Verification items for the finished model (mm, model axes). A direction names the side the tool comes from. Coordinates: 2 decimals unless noted, no trailing zeros. Order: outer loops, then holes, each group sorted by start corner. A loop starts at its lowest first (then second) coordinate and runs counter-clockwise, first axis right, second up. Notation, with made-up numbers: M -7.5,-0.75 L 37.5,-0.75 A33 cw 37.5,28.25 Z; hole C 77,5 d2. An arc over 180 degrees is marked long. Return JSON: item names as keys, results as strings. Group by question number.
Q1. Section check B-B, the plane x = 0. Enter the section's corners in (y, z).
Q2. Mould release check, pull along Z, two halves, no side actions. Record for faces 1 (the face through (-10.4, 10.922, -6.3)), 2 (the face through (-9.37, 15.93, -7.19)), 3 (the face through (0, 11, 2.699)): pulls with the +Z half, pulls with the -Z half, needs draft (parallel to the pull), parting line crosses it, or undercut.
Q3. Thickness scan on probe 1 along Z at (x, y) = (0, 1.95); probe 2 along X at (y, z) = (2.75, -13); probe 3 along Y at (x, z) = (11.5, -20.5). Record the ranges inside material, lowest first.
Q4. Section check C-C, the plane y = 1.5. Enter the section's corners in (x, z), then the cut area to 3 significant figures.
Q5. Section check D-D, the plane x = 13. Enter the section's corners in (y, z), then the cut area to 3 significant figures.
Q6. Access from +Z, -Z, +X, -X, +Y, -Y to the whole of each face (thin tool, end or side, straight path). Record for faces 4 (the face through (0, 21.082, -3)), 5 (the face through (-1.82, 7.96, 13.85)), 6 (the face through (0, 11, -2.699)).
Q7. Go/stop test with flat-tipped pins: pin 1 Ø6.5 at (x, z) = (-20.62, -11.91) entering from +Y; pin 2 Ø3 at (y, z) = (10.5, 9) entering from +X; pin 3 Ø5 at (y, z) = (9, 2) entering from +X. Record where each tip stops, or that it passes through.
Q8. Section check A-A, the plane y = 5.75. Enter the section's corners in (x, z).
Autodesk Inventor part; units mm, degrees
ref_plane "YZ Plane" through (0, 0, 0) normal (1, 0, 0) x (0, 1, 0)
ref_plane "XZ Plane" through (0, 0, 0) normal (0, 1, 0) x (-1, 0, 0)
ref_plane "XY Plane" through (0, 0, 0) normal (0, 0, 1) x (1, 0, 0)
sketch "Sketch1" plane through (0, 0, 0) normal (0, 1, 0) x (-1, 0, 0)
  circle A0 centre (0, 0) radius 27.94
  dimension "d0" = 55.88
extrude "Extrusion1" add sketch "Sketch1" along normal blind 5.08
sketch "Sketch2" plane through (0, 5.08, 0) normal (0, 1, 0) x (1, 0, 0)
  circle A0 centre (0, 0) radius 13.97
  dimension "d3" = 27.94
extrude "Extrusion2" add sketch "Sketch2" along normal blind 5.842
sketch "Sketch3" plane through (0, 10.922, 0) normal (0, 1, 0) x (1, 0, 0)
  circle A0 centre (0, 0) radius 11.811
  dimension "d6" = 23.622
extrude "Extrusion3" add sketch "Sketch3" along normal blind 10.16
sketch "Sketch5" plane through (0, 21.082, 0) normal (0, 1, 0) x (1, 0, 0)
  line L0 (0, 0) -> (0, 2.667)
  line L1 (-3.1168, 0) -> (-1.5584, 2.6992)
  line L2 (-1.5584, 2.6992) -> (1.5584, 2.6992)
  line L3 (1.5584, 2.6992) -> (3.1168, 0)
  line L4 (3.1168, 0) -> (1.5584, -2.6992)
  line L5 (1.5584, -2.6992) -> (-1.5584, -2.6992)
  line L6 (-1.5584, -2.6992) -> (-3.1168, 0)
  dimension "d10" = 2.667
extrude "Extrusion4" cut sketch "Sketch5" against normal blind 25.4
sketch "Sketch6" plane through (0, 5.08, 0) normal (0, 1, 0) x (1, 0, 0)
  circle A0 centre (0, 0) radius 27.94
  circle A1 centre (0, 23.8125) radius 1.9939
  circle A2 centre (20.6222, 11.9063) radius 1.9939
  circle A3 centre (20.6222, -11.9063) radius 1.9939
  circle A4 centre (0, -23.8125) radius 1.9939
  circle A5 centre (-20.6222, -11.9063) radius 1.9939
  circle A6 centre (-20.6222, 11.9063) radius 1.9939
extrude "Extrusion5" cut sketch "Sketch6" against normal blind 25.4 contours A1 | A2 | A3 | A4 | A5 | A6
properties part number "Wheel Mount"
Numbers:
{
 "1": {"outline": "M 0,-27.94 L 5.08,-27.94 L 5.08,-25.81 L 0,-25.81 Z; M 0,-21.82 L 5.08,-21.82 L 5.08,-13.97 L 10.92,-13.97 L 10.92,-11.81 L 21.08,-11.81 L 21.08,-2.7 L 0,-2.7 Z; M 0,2.7 L 21.08,2.7 L 21.08,11.81 L 10.92,11.81 L 10.92,13.97 L 5.08,13.97 L 5.08,21.82 L 0,21.82 Z; M 0,25.81 L 5.08,25.81 L 5.08,27.94 L 0,27.94 Z"},
 "2": {"face 1": "needs draft", "face 2": "parting line crosses it", "face 3": "undercut"},
 "3": {"probe 1": "z = -27.94 to -25.81, -21.82 to -2.7, 2.7 to 21.82, 25.81 to 27.94", "probe 2": "x = -24.73 to -22.29, -18.96 to 18.96, 22.29 to 24.73", "probe 3": "y = 0 to 5.08"},
 "4": {"outline": "C 0,0 d55.88; hole C -20.62,-11.91 d3.99; hole C -20.62,11.91 d3.99; hole M -3.12,0 L -1.56,-2.7 L 1.56,-2.7 L 3.12,0 L 1.56,2.7 L -1.56,2.7 Z; hole C 0,-23.81 d3.99; hole C 0,23.81 d3.99; hole C 20.62,-11.91 d3.99; hole C 20.62,11.91 d3.99", "area": "2,350 mm2"},
 "5": {"outline": "M 0,-24.73 L 5.08,-24.73 L 5.08,-5.11 L 10.92,-5.11 L 10.92,5.11 L 5.08,5.11 L 5.08,24.73 L 0,24.73 Z", "area": "311 mm2"},
 "6": {"face 4": "+Z, -Z, +X, -X, +Y", "face 5": "+Y", "face 6": "+Y, -Y"},
 "7": {"pin 1": "stops at y = 5.08", "pin 2": "stops at x = 11.79", "pin 3": "stops at x = 13.97"},
 "8": {"outline": "C 0,0 d27.94; hole M -3.12,0 L -1.56,-2.7 L 1.56,-2.7 L 3.12,0 L 1.56,2.7 L -1.56,2.7 Z"}
}
